```python
from build123d import *

# Parameters (mm, degrees)
SKETCH_R  = 1.5
PAD_DEPTH = 1.8542


with BuildPart() as part:
    # Sketch (on Face48 of Binder001) → Pad (new body)
    with BuildSketch(Plane.YZ.offset(326.1082)):
        with BuildLine():
            Line((129.0813, -24.706), (127.2271, -24.706))
            ThreePointArc((127.2271, -24.706), (126.378572, -25.057472), (126.0271, -25.906))
            Line((126.0271, -86.594), (126.0271, -25.906))
            ThreePointArc((126.0271, -86.594), (126.378572, -87.442528), (127.2271, -87.794))
            Line((129.0813, -87.794), (127.2271, -87.794))
            ThreePointArc((130.2813, -88.994), (129.929828, -88.145472), (129.0813, -87.794))
            Line((130.2813, -88.994), (130.2813, -101.3746))
            ThreePointArc((130.2813, -101.3746), (130.632772, -102.223128), (131.4813, -102.5746))
            Line((131.4813, -102.5746), (176.6813, -102.5746))
            ThreePointArc((176.6813, -102.5746), (177.529828, -102.223128), (177.8813, -101.3746))
            Line((177.8813, -88.994), (177.8813, -101.3746))
            ThreePointArc((179.0813, -87.794), (178.232772, -88.145472), (177.8813, -88.994))
            Line((180.9355, -87.794), (179.0813, -87.794))
            ThreePointArc((180.9355, -87.794), (181.784028, -87.442528), (182.1355, -86.594))
            Line((182.1355, -25.906), (182.1355, -86.594))
            ThreePointArc((182.1355, -25.906), (181.784028, -25.057472), (180.9355, -24.706))
            Line((179.0813, -24.706), (180.9355, -24.706))
            ThreePointArc((177.8813, -23.506), (178.232772, -24.354528), (179.0813, -24.706))
            Line((177.8813, -11.1254), (177.8813, -23.506))
            ThreePointArc((177.8813, -11.1254), (177.529828, -10.276872), (176.6813, -9.9254))
            Line((131.4813, -9.9254), (176.6813, -9.9254))
            ThreePointArc((131.4813, -9.9254), (130.632772, -10.276872), (130.2813, -11.1254))
            Line((130.2813, -11.1254), (130.2813, -23.506))
            ThreePointArc((129.0813, -24.706), (129.929828, -24.354528), (130.2813, -23.506))
        make_face()
        with Locations((134.0813, -56.25)):
            Circle(SKETCH_R, mode=Mode.SUBTRACT)
        with Locations((174.0813, -56.25)):
            Circle(SKETCH_R, mode=Mode.SUBTRACT)
        with BuildLine():
            Line((139.9043, -22.5), (139.9043, -90))
            ThreePointArc((139.9043, -90), (140.67373, -91.85757), (142.5313, -92.627))
            Line((142.5313, -92.627), (165.6313, -92.627))
            ThreePointArc((165.6313, -92.627), (167.48887, -91.85757), (168.2583, -90))
            Line((168.2583, -90), (168.2583, -22.5))
            ThreePointArc((168.2583, -22.5), (167.48887, -20.64243), (165.6313, -19.873))
            Line((165.6313, -19.873), (142.5313, -19.873))
            ThreePointArc((142.5313, -19.873), (140.67373, -20.64243), (139.9043, -22.5))
        make_face(mode=Mode.SUBTRACT)
        with BuildLine():
            ThreePointArc((133.4436, -12.0336), (132.3895, -13.0877), (133.4436, -14.1418))
            Line((133.4436, -14.1418), (174.719, -14.1418))
            ThreePointArc((174.719, -14.1418), (175.7731, -13.0877), (174.719, -12.0336))
            Line((133.4436, -12.0336), (174.719, -12.0336))
        make_face(mode=Mode.SUBTRACT)
        with BuildLine():
            ThreePointArc((133.4436, -98.3582), (132.3895, -99.4123), (133.4436, -100.4664))
            Line((133.4436, -100.4664), (174.719, -100.4664))
            ThreePointArc((174.719, -100.4664), (175.7731, -99.4123), (174.719, -98.3582))
            Line((133.4436, -98.3582), (174.719, -98.3582))
        make_face(mode=Mode.SUBTRACT)
    extrude(amount=PAD_DEPTH)


solid = part.part
```
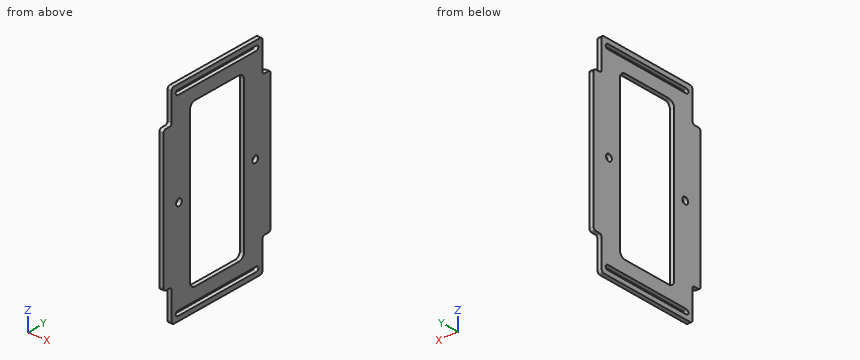
Geometry check sheet. Reference: the model listing, model coordinates, mm. Give positions to 0.01 mm unless a question says otherwise; leave off trailing zeros. Loops run counter-clockwise (first coordinate to the right, second up) from the corner with the lowest first, then second, coordinate; pieces in that order, holes last. Notation, with made-up numbers: M 79.25,-15.5 L 107.25,-15.5 A14 ccw 107.25,-6.5 Z; hole C -1.5,64.5 d10. An arc over 180 degrees is marked long. Write item = value, one per line.
(1) Sectioned sample at A-A, the plane y = 170.5. Record the cut outline in (x, z), plus the area to 3 significant figures.
Answer below:
outline = M 326.11,-102.57 L 327.96,-102.57 L 327.96,-100.47 L 326.11,-100.47 Z; M 326.11,-98.36 L 327.96,-98.36 L 327.96,-14.14 L 326.11,-14.14 Z; M 326.11,-12.03 L 327.96,-12.03 L 327.96,-9.93 L 326.11,-9.93 Z
area = 164 mm2
(2) Material ranges on line 1 (Z direction, x = 327.8, y = 149); line 2 (Y direction, x = 326.4, z = -59); line 3 (Z direction, x = 326.95, y = 171.5), recorded low to high. Write a range as [from, to].
Answer below:
line_1 = [-102.57, -100.47], [-98.36, -92.63], [-19.87, -14.14], [-12.03, -9.93]
line_2 = [126.03, 139.9], [168.26, 182.14]
line_3 = [-102.57, -100.47], [-98.36, -14.14], [-12.03, -9.93]
(3) Sectioned sample at C-C, the plane y = 158.5. Record the cut outline in (x, z).
Answer below:
outline = M 326.11,-102.57 L 327.96,-102.57 L 327.96,-100.47 L 326.11,-100.47 Z; M 326.11,-98.36 L 327.96,-98.36 L 327.96,-92.63 L 326.11,-92.63 Z; M 326.11,-19.87 L 327.96,-19.87 L 327.96,-14.14 L 326.11,-14.14 Z; M 326.11,-12.03 L 327.96,-12.03 L 327.96,-9.93 L 326.11,-9.93 Z
(4) Sectioned sample at D-D, the plane x = 327.25. State how many separate pieces and enclosed holes the cut face has, plus the area to 3 significant figures.
Answer below:
separate_pieces = 1
enclosed_holes = 5
area = 2,690 mm2
(5) Sectioned sample at B-B, the plane z = -56.25. Record the cut outline in (x, y).
Answer below:
outline = M 326.11,126.03 L 327.96,126.03 L 327.96,132.58 L 326.11,132.58 Z; M 326.11,135.58 L 327.96,135.58 L 327.96,139.9 L 326.11,139.9 Z; M 326.11,168.26 L 327.96,168.26 L 327.96,172.58 L 326.11,172.58 Z; M 326.11,175.58 L 327.96,175.58 L 327.96,182.14 L 326.11,182.14 Z
(6) Gauge pin test, flat ends, axial feed: pin 1 Ø5 at (y, z) = (165.5, -51) entering from -X; pin 2 Ø0.6 at (x, z) = (327.5, -15.5) entering from +Y. Record the tip position at first contact, or that the pin passes through.
Answer below:
pin_1 = through
pin_2 = 177.88
